```python
from build123d import *

# Parameters (mm, degrees)
CROQUIS1_R               = 20
CROQUIS1_R_2             = 17
REVOLUCI_N_L_MINA1_ANGLE = 90
CROQUIS3_R               = 20
CROQUIS3_R_2             = 17
EXTRUIR1_DEPTH           = 18
CROQUIS4_R               = 20
CROQUIS4_R_2             = 17
EXTRUIR2_DEPTH           = 18
REDONDEO1_R              = 1


with BuildPart() as part:
    # Croquis1 → Revolución-Lámina1 (revolve)
    with BuildSketch(Plane(origin=(0, 0, 0), x_dir=(0, 0, -1), z_dir=(1, 0, 0))):
        with Locations((-21, 0)):
            Circle(CROQUIS1_R)
        with Locations((-21, 0)):
            Circle(CROQUIS1_R_2, mode=Mode.SUBTRACT)
    revolve(axis=Axis((0, 0, 0), (0, 1, 0)), revolution_arc=REVOLUCI_N_L_MINA1_ANGLE)

    # Croquis3 → Extruir1 (add)
    with BuildSketch(Plane.ZY):
        with Locations((21, 0)):
            Circle(CROQUIS3_R)
        with Locations((21, 0)):
            Circle(CROQUIS3_R_2, mode=Mode.SUBTRACT)
    extrude(amount=EXTRUIR1_DEPTH)

    # Croquis4 → Extruir2 (add)
    with BuildSketch(Plane(origin=(0, 0, 0), x_dir=(-1, 0, 0), z_dir=(0, 0, -1))):
        with Locations(Location((-21, 0, 0), (0, 0, 180))):
            Circle(CROQUIS4_R)
        with Locations(Location((-21, 0, 0), (0, 0, 180))):
            Circle(CROQUIS4_R_2, mode=Mode.SUBTRACT)
    extrude(amount=EXTRUIR2_DEPTH)

    # Redondeo1
    redondeo1_edges = [part.edges().sort_by_distance(p)[0] for p in [
        (1, 0, -18),
        (-18, 0, 1),
    ]]
    fillet(redondeo1_edges, radius=REDONDEO1_R)


solid = part.part
```
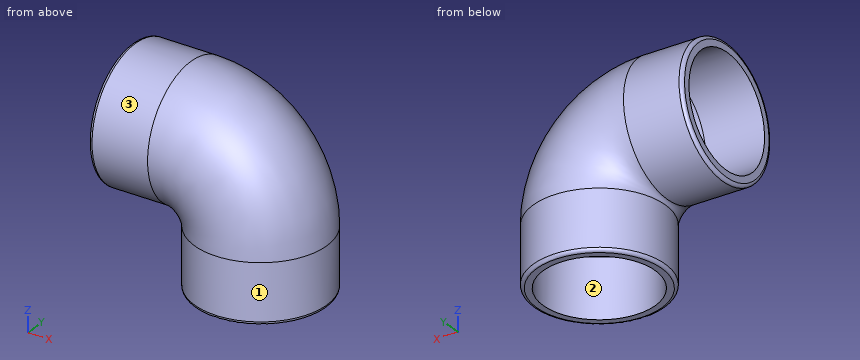
The listing builds one solid part. Answer for the finished solid, in the listing's coordinates (mm). Face numbers are marked on the shaded views. Give positions to 0.01 mm unless a question says otherwise; leave off trailing zeros. Order: outer loops, then holes, each group sorted by start corner. A loop starts at its lowest first (then second) coordinate and runs counter-clockwise, first axis right, second up. Notation, with made-up numbers: (8, 22) -> (32, 22) arc R14 ccw to (32, 35) -> close; hole circle Ø5 at (-38.75, 75). An arc over 180 degrees is marked (long way). One line per item, written item: value.
1) Find section A-A, the plane y = 0. Determine the outline of the cut face in (x, z).
Reported:
outline: (-18, 2) arc R1 ccw to (-17, 1) -> (0, 1) arc R1 cw to (1, 0) -> (1, -17) arc R1 ccw to (2, -18) -> (4, -18) -> (4, 0) arc R4 ccw to (0, 4) -> (-18, 4) -> close; (-18, 38) -> (0, 38) arc R38 cw to (38, 0) -> (38, -18) -> (40, -18) arc R1 ccw to (41, -17) -> (41, 0) arc R41 ccw to (0, 41) -> (-17, 41) arc R1 ccw to (-18, 40) -> close
2) Find section B-B, the plane z = -8.5. Determine the outline of the cut face in (x, y).
Reported:
outline: circle Ø40 at (21, 0); hole circle Ø34 at (21, 0)
3) Find the intervals of material crossed by line 1 (Y direction, x = 21, z = -9); line 2 (Z direction, x = -13.75, y = 0); line 3 (Y direction, x = 10, z = -11), in increasing order.
Reported:
line 1: y = -20 to -17, 17 to 20
line 2: z = 1 to 4, 38 to 41
line 3: y = -16.7 to -12.96, 12.96 to 16.7
4) Find section C-C, the plane x = -7.5. Determine the outline of the cut face in (y, z), plus the area to 3 significant figures.
Reported:
outline: circle Ø40 at (0, 21); hole circle Ø34 at (0, 21)
area: 349 mm^2
5) Flat-ended cylindrical pins translate along their axes: P1, Ø12, axis at y = -4.5, z = 10.5, coming from the -X side; P2, Ø10, axis at x = -11.5, z = 7.5, coming from the -Y side; P3, Ø5, axis at x = -9, y = -6, coming from the +Z side; P4, Ø4, axis at x = 1, y = -15.5, coming from the -Z side. Find the tip coordinate at first contact, or state that the pin passes through.
Reported:
P1: stops at x = -18
P2: stops at y = -18.1
P3: stops at z = 40.69
P4: stops at z = 6.12
6) Determine the mould class of the marked faces 1, 2 and 3 for opening direction X: pulls with the +X half, pulls with the -X half, needs draft (parallel to the pull), parting line crosses it, or undercut.
Reported:
face 1: parting line crosses it
face 2: undercut
face 3: needs draft
